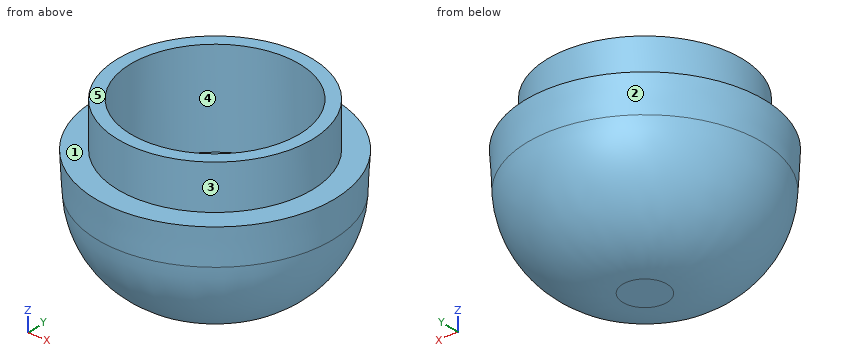
```python
from build123d import *

# Parameters (mm, degrees)
SKETCH1_R           = 4.7625
BASE_EXTRUDE_DEPTH  = 5.08
BASE_EXTRUDE_DRAFT  = -3
FILLET3_R           = 3.81
SKETCH2_R           = 3.8735
BOSS_EXTRUDE1_DEPTH = 1.778
SKETCH3_R           = 3.3655
CUT_EXTRUDE1_DEPTH  = 3.81


with BuildPart() as part:
    # Sketch1 → Base-Extrude (with draft: the straight prism first)
    with BuildSketch(Plane.XY):
        Circle(SKETCH1_R)
    extrude(amount=-BASE_EXTRUDE_DEPTH)
    # Base-Extrude: the draft: its side faces are tilted about the plane it starts from
    base_extrude_sides = [part.faces().sort_by_distance(p)[0] for p in [
        (-4.7625, 0, -2.54),
    ]]
    draft(base_extrude_sides, Plane.XY, BASE_EXTRUDE_DRAFT)

    # Fillet3
    fillet3_edges = [part.edges().sort_by_distance(p)[0] for p in [
        (-4.496268481, 0, -5.08),
    ]]
    fillet(fillet3_edges, radius=FILLET3_R)

    # Sketch2 → Boss-Extrude1 (add)
    with BuildSketch(Plane.XY):
        Circle(SKETCH2_R)
    extrude(amount=BOSS_EXTRUDE1_DEPTH)

    # Sketch3 → Cut-Extrude1 (cut)
    with BuildSketch(Plane.XY.offset(1.778)):
        Circle(SKETCH3_R)
    extrude(amount=-CUT_EXTRUDE1_DEPTH, mode=Mode.SUBTRACT)


solid = part.part
```
Work out the finished part from the listing and answer in its coordinate system (mm). Face numbers are marked on the shaded views. A direction names the side the tool comes from. Round coordinates to 2 decimals unless told otherwise and drop trailing zeros. Order: outer loops, then holes, each group sorted by start corner. A loop starts at its lowest first (then second) coordinate and runs counter-clockwise, first axis right, second up.
Q1. Find the intervals of material crossed by line 1 along Y through (x, z) = (0, 0.95); line 2 along Y through (x, z) = (0, -0.3); line 3 along X through (y, z) = (-1.5, -1.75), in increasing order.
Solution:
line 1: y = -3.87 to -3.37, 3.37 to 3.87
line 2: y = -4.75 to -3.37, 3.37 to 4.75
line 3: x = -4.41 to -3.01, 3.01 to 4.41
Q2. A cutting plane is placed at A-A, the plane z = 0.25. Determine the outline of the cut face in (x, y).
Solution:
outline: circle Ø7.75 at (0, 0); hole circle Ø6.73 at (0, 0)
Q3. A tool of negligible diameter and unlimited length cuts with its end or side. For the marked faces 1 and 2, from which of +Z, -Z, +X, -X, +Y, -Y can it reach the whole face along a straight path? Write none if from no direction.
Solution:
face 1: +Z
face 2: -Z
Q4. Given pin 1 Ø4 at (x, z) = (-1, -3.5) entering from +Y; pin 2 Ø1.5 at (x, y) = (-2, 0.5) entering from +Z; pin 3 Ø2 at (y, z) = (2.5, -3) entering from -X, each flat-ended and moving along its own axis, determine where each tip first touches the part or whether it passes through.
Solution:
pin 1: stops at y = 4.67
pin 2: stops at z = -2.03
pin 3: stops at x = -4.19
Q5. The mould has two halves that part along Y. Classify the marked faces 3, 4 and 5: pulls with the +Y half, pulls with the -Y half, needs draft (parallel to the pull), parting line crosses it, or undercut.
Solution:
face 3: parting line crosses it
face 4: undercut
face 5: needs draft
